Geometry: see drawing. Coordinates: mm, zero at the bounding-box minimum. Coordinates: 2 decimals unless noted, no trailing zeros. Order: outer loops, then holes, each group sorted by start corner. A loop starts at its lowest first (then second) coordinate and runs counter-clockwise, first axis right, second up.
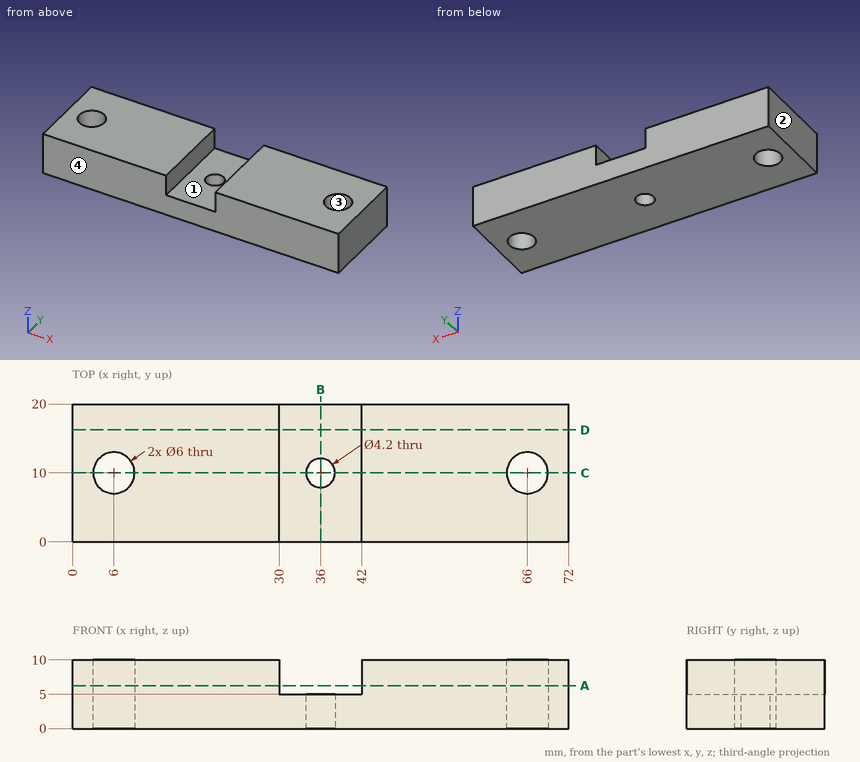
Item 1: Ray query, probe 1 along Y at (x, z) = (6, 6); probe 2 along X at (y, z) = (18.25, 8.75); probe 3 along X at (y, z) = (8.25, 3.5). Return the intervals inside material, ascending.
Response values:
probe 1: y = 0 to 7, 13 to 20
probe 2: x = 0 to 30, 42 to 72
probe 3: x = 0 to 3.56, 8.44 to 34.84, 37.16 to 63.56, 68.44 to 72
Item 2: Cut plane B-B on x = 36. Return loops of the section in (y, z), then the cut area to 3 significant figures.
Response values:
outline: (0, 0) - (7.9, 0) - (7.9, 5) - (0, 5) - close; (12.1, 0) - (20, 0) - (20, 5) - (12.1, 5) - close
area: 79.0 mm2
Item 3: Cut plane A-A on z = 6.25. Return loops of the section in (x, y).
Response values:
outline: (0, 0) - (30, 0) - (30, 20) - (0, 20) - close; (42, 0) - (72, 0) - (72, 20) - (42, 20) - close; hole circle Ø6 at (6, 10); hole circle Ø6 at (66, 10)
Item 4: Pin query (flat end, axial travel): pin 1 Ø1 at (x, z) = (52.5, 6) entering from -Y; pin 2 Ø3.5 at (x, y) = (66, 10) entering from +Z. Return the tip coordinate at first contact, or that it passes through.
Response values:
pin 1: stops at y = 0
pin 2: passes through
Item 5: Draft query along X for the marked faces 1, 2, 3 and 4. Return one class per face: pulls with the +X half, pulls with the -X half, needs draft (parallel to the pull), parting line crosses it, or undercut.
Response values:
face 1: undercut
face 2: pulls with the -X half
face 3: undercut
face 4: needs draft
Item 6: Cut plane D-D on y = 16.25. Return loops of the section in (x, z).
Response values:
outline: (0, 0) - (72, 0) - (72, 10) - (42, 10) - (42, 5) - (30, 5) - (30, 10) - (0, 10) - close
Item 7: Cut plane C-C on y = 10. Return loops of the section in (x, z).
Response values:
outline: (0, 0) - (3, 0) - (3, 10) - (0, 10) - close; (9, 0) - (33.9, 0) - (33.9, 5) - (30, 5) - (30, 10) - (9, 10) - close; (38.1, 0) - (63, 0) - (63, 10) - (42, 10) - (42, 5) - (38.1, 5) - close; (69, 0) - (72, 0) - (72, 10) - (69, 10) - close
